```python
from build123d import *
from OCP.BRepFilletAPI import BRepFilletAPI_MakeChamfer

# Parameters (mm, degrees)
SKETCH1_R                   = 15.875
EXTRUDE1_DEPTH              = 6.35
CHAMFER1_SIZE               = 2.286
CHAMFER1_SIZE2              = 8.531468146
F_1_4_CLEARANCE_HOLE1_D     = 7.14248
F_1_4_20_TAPPED_HOLE1_D     = 5.1054
F_1_4_20_TAPPED_HOLE1_DEPTH = 16.51
F_1_4_20_TAPPED_HOLE1_TIP   = 1.533816902
FILLET1_R                   = 19.05


with BuildPart() as part:
    # Sketch1 → Extrude1 (new body)
    with BuildSketch(Plane.XY):
        with BuildLine():
            Line((0, 0), (0, -19.05))
            Line((0, -19.05), (39.953569803, -19.05))
            ThreePointArc((39.953569803, -19.05), (63.5, -34.925), (87.046430197, -19.05))
            Line((87.046430197, -19.05), (127, -19.05))
            Line((127, -19.05), (127, 0))
            Line((127, 0), (87.046430197, 0))
            ThreePointArc((87.046430197, 0), (63.5, 15.875), (39.953569803, 0))
            Line((39.953569803, 0), (0, 0))
        make_face()
        with Locations((63.5, -9.525)):
            Circle(SKETCH1_R, mode=Mode.SUBTRACT)
    extrude(amount=EXTRUDE1_DEPTH)

    # Chamfer1: one chamfer whose edges measure the first distance from different faces: ONE call of the kernel's chamfer builder (chamfer() names one face for all edges)
    chamfer1_edges_1 = [part.edges().sort_by_distance(p)[0] for p in [
        (127, 0, 3.175),
    ]]
    chamfer1_side_1 = [part.faces().sort_by_distance(p)[0] for p in [
        (107.023215098, 0, 3.175),
    ]]
    chamfer1_edges_2 = [part.edges().sort_by_distance(p)[0] for p in [
        (127, -19.05, 3.175),
    ]]
    chamfer1_side_2 = [part.faces().sort_by_distance(p)[0] for p in [
        (107.023215098, -19.05, 3.175),
    ]]
    chamfer1_edges_3 = [part.edges().sort_by_distance(p)[0] for p in [
        (0, -19.05, 3.175),
    ]]
    chamfer1_side_3 = [part.faces().sort_by_distance(p)[0] for p in [
        (19.976784902, -19.05, 3.175),
    ]]
    chamfer1_edges_4 = [part.edges().sort_by_distance(p)[0] for p in [
        (0, 0, 3.175),
    ]]
    chamfer1_side_4 = [part.faces().sort_by_distance(p)[0] for p in [
        (19.976784902, 0, 3.175),
    ]]
    chamfer1 = BRepFilletAPI_MakeChamfer(part.part.solid().wrapped)
    for e in chamfer1_edges_1:
        chamfer1.Add(CHAMFER1_SIZE, CHAMFER1_SIZE2, e.wrapped, chamfer1_side_1[0].wrapped)  # the first distance lies on this face
    for e in chamfer1_edges_2:
        chamfer1.Add(CHAMFER1_SIZE, CHAMFER1_SIZE2, e.wrapped, chamfer1_side_2[0].wrapped)  # the first distance lies on this face
    for e in chamfer1_edges_3:
        chamfer1.Add(CHAMFER1_SIZE, CHAMFER1_SIZE2, e.wrapped, chamfer1_side_3[0].wrapped)  # the first distance lies on this face
    for e in chamfer1_edges_4:
        chamfer1.Add(CHAMFER1_SIZE, CHAMFER1_SIZE2, e.wrapped, chamfer1_side_4[0].wrapped)  # the first distance lies on this face
    add(Compound.cast(chamfer1.Shape()), mode=Mode.REPLACE)

    # 1/4 Clearance Hole1 (through all)
    with Locations(Plane(origin=(6.35, -9.525, 6.35), x_dir=(1, 0, 0), z_dir=(0, 0, 1))):
        with Locations((0, 0), (114.3, 0)):
            Hole(F_1_4_CLEARANCE_HOLE1_D / 2)

    # 1/4-20 Tapped Hole1
    with Locations(Plane(origin=(40.64, -9.525, 0), x_dir=(-1, 0, 0), z_dir=(0, 0, -1))):
        with Locations((0, 0), (-45.72, 0)):
            Hole(F_1_4_20_TAPPED_HOLE1_D / 2, depth=F_1_4_20_TAPPED_HOLE1_DEPTH)
            with Locations((0, 0, -(F_1_4_20_TAPPED_HOLE1_DEPTH + F_1_4_20_TAPPED_HOLE1_TIP / 2))):  # 118° drill point
                Cone(0, F_1_4_20_TAPPED_HOLE1_D / 2, F_1_4_20_TAPPED_HOLE1_TIP, mode=Mode.SUBTRACT)

    # Fillet1
    fillet1_edges = [part.edges().sort_by_distance(p)[0] for p in [
        (39.953569803, 0, 3.175),
        (87.046430197, 0, 3.175),
        (87.046430197, -19.05, 3.175),
        (39.953569803, -19.05, 3.175),
    ]]
    fillet(fillet1_edges, radius=FILLET1_R)


solid = part.part
```
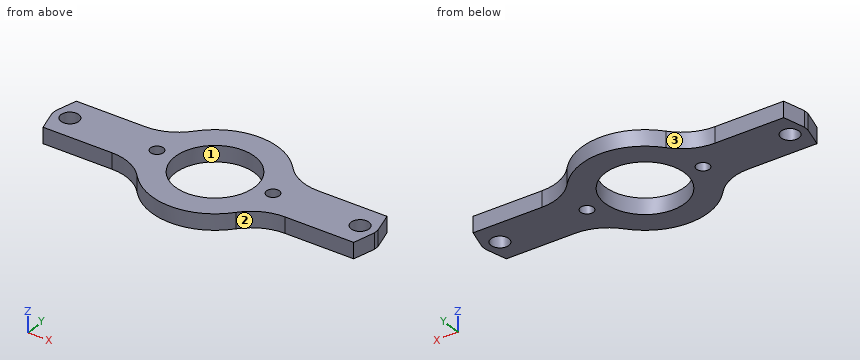
The model under review builds one solid part; all positions refer to its coordinate system, in mm. Face numbers are marked on the shaded views. Give positions to 0.01 mm unless a question says otherwise; leave off trailing zeros. Loops run counter-clockwise (first coordinate to the right, second up) from the corner with the lowest first, then second, coordinate; pieces in that order, holes last. Notation, with made-up numbers: (82.25, 86.25) - (135.25, 86.25) arc R21 cw to (135.25, 120.25) - close; hole circle Ø8 at (34, 32). An arc over 180 degrees is marked (long way). Answer as a JSON object with one key per item and string values.
Q1. Mouldability with a two-part tool opening along Y and no side actions: class the marked faces 1, 2 and 3 as +Y half, -Y half, draft (parallel to the pull), parting line (faces both ways), or undercut.
Worked out:
{"face 1": "undercut", "face 2": "-Y half", "face 3": "+Y half"}
Q2. Add section C-C on z = 4.75. State the section outline as (x, y) points (3 decimals).
Worked out:
{"outline": "(0, -10.519) - (2.286, -19.05) - (29.452, -19.05) arc R19.05 cw to (44.044, -25.854) arc R25.4 ccw to (82.956, -25.854) arc R19.05 cw to (97.548, -19.05) - (124.714, -19.05) - (127, -10.519) - (127, -8.531) - (124.714, 0) - (97.548, 0) arc R19.05 cw to (82.956, 6.804) arc R25.4 ccw to (44.044, 6.804) arc R19.05 cw to (29.452, 0) - (2.286, 0) - (0, -8.531) - close; hole circle Ø7.142 at (6.35, -9.525); hole circle Ø5.105 at (40.64, -9.525); hole circle Ø31.75 at (63.5, -9.525); hole circle Ø5.105 at (86.36, -9.525); hole circle Ø7.142 at (120.65, -9.525)"}
Q3. Insertion check: pin 1 (1.9 mm diameter, centred on x = 14.5, z = 1.5, fed in from +Y); pin 2 (3 mm diameter, centred on x = 12.5, z = 3, fed in from -Y); pin 3 (1 mm diameter, centred on y = -22, z = 4, fed in from +X). Each pin has a flat end and moves straight along its axis. Give the tip position at first contact, or say it passes through.
Worked out:
{"pin 1": "stops at y = 0", "pin 2": "stops at y = -19.05", "pin 3": "stops at x = 88.2"}
Q4. Add section B-B on x = 63.5. State the section outline as (y, z) points (3 decimals).
Worked out:
{"outline": "(-34.925, 0) - (-25.4, 0) - (-25.4, 6.35) - (-34.925, 6.35) - close; (6.35, 0) - (15.875, 0) - (15.875, 6.35) - (6.35, 6.35) - close"}
Q5. Add section A-A on x = 120.65. State the section outline as (y, z) points, plus the area to 3 significant figures.
Worked out:
{"outline": "(-19.05, 0) - (-13.1, 0) - (-13.1, 6.35) - (-19.05, 6.35) - close; (-5.95, 0) - (0, 0) - (0, 6.35) - (-5.95, 6.35) - close", "area": "75.6 mm^2"}
Q6. To check wall thickness, follow line 1 along Y through (x, z) = (120.65, 1.5); line 2 along X through (y, z) = (-12.5, 5.75); line 3 along X through (y, z) = (-8.5, 1.75). State the ranges of each line that lie inside material, in increasing order.
Worked out:
{"line 1": "y = -19.05 to -13.1, -5.95 to 0", "line 2": "x = 0.53 to 4.37, 8.33 to 47.91, 79.09 to 118.67, 122.63 to 126.47", "line 3": "x = 0.01 to 2.93, 9.77 to 38.3, 42.98 to 47.66, 79.34 to 84.02, 88.7 to 117.23, 124.07 to 126.99"}
